```python
from build123d import *

# Parameters (mm, degrees)
F0_W     = 44.45
F0_H     = 44.45
F1_DEPTH = 19.05
F2_R     = 2.38125
F3_DEPTH = 44.451
F2_R_2   = 3.96875
F4_DEPTH = 3.81


with BuildPart() as f1:
    # F0 (on Front) → F1 (new body, symmetric)
    with BuildSketch(Plane.XZ):
        Rectangle(F0_W, F0_H)
    extrude(amount=F1_DEPTH, both=True)

    # F2 (on face) → F3 (cut, through all)
    with BuildSketch(Plane(origin=(0, 0, -22.225), x_dir=(1, 0, 0), z_dir=(0, 0, -1))):
        Circle(F2_R)
    extrude(amount=-F3_DEPTH, mode=Mode.SUBTRACT)

    # F2 (on face) → F4 (cut)
    with BuildSketch(Plane(origin=(0, 0, -22.225), x_dir=(1, 0, 0), z_dir=(0, 0, -1))):
        Circle(F2_R_2)
        Circle(F2_R, mode=Mode.SUBTRACT)
    extrude(amount=-F4_DEPTH, mode=Mode.SUBTRACT)


solid = f1.part
```
For this review, take the finished solid that the model builds, in its own axes (mm). A direction names the side the tool comes from. Round coordinates to 2 decimals unless told otherwise and drop trailing zeros. Loops run counter-clockwise (first coordinate to the right, second up) from the corner with the lowest first, then second, coordinate; pieces in that order, holes last.
(1) Tool access review of faces 4 (the flat face through (2, 2, -18.415)), 5 (the cylindrical face through (-1.89, 1.45, 1.62)): name each direction out of +Z, -Z, +X, -X, +Y, -Y from which nothing blocks a thin tool from reaching the whole face with its end or side.
Returned:
face 4: -Z
face 5: +Z, -Z
(2) We need section A-A (x = 0). Give the boundary of the cut face in (y, z) (3 decimals).
Returned:
outline: (-19.05, -22.225) - (-3.969, -22.225) - (-3.969, -18.415) - (-2.381, -18.415) - (-2.381, 22.225) - (-19.05, 22.225) - close; (2.381, -18.415) - (3.969, -18.415) - (3.969, -22.225) - (19.05, -22.225) - (19.05, 22.225) - (2.381, 22.225) - close
(3) We need section B-B (y = 0). Give the boundary of the cut face in (x, z) (3 decimals), plus the area to 3 significant figures.
Returned:
outline: (-22.225, -22.225) - (-3.969, -22.225) - (-3.969, -18.415) - (-2.381, -18.415) - (-2.381, 22.225) - (-22.225, 22.225) - close; (2.381, -18.415) - (3.969, -18.415) - (3.969, -22.225) - (22.225, -22.225) - (22.225, 22.225) - (2.381, 22.225) - close
area: 1,750 mm2
(4) Wall thickness on line 1 along Y through (x, z) = (0, -8); line 2 along Y through (x, z) = (0, -21); line 3 along X through (y, z) = (0, 5) (3 decimals): over which ranges is each line inside the solid? List them lowest first.
Returned:
line 1: y = -19.05 to -2.38, 2.38 to 19.05
line 2: y = -19.05 to -3.97, 3.97 to 19.05
line 3: x = -22.225 to -2.381, 2.381 to 22.225
(5) Clearance check with flat-ended pins moving along their axes: P1, Ø2.5, axis at x = -2, y = -2, coming from the -Z side (3 decimals); P2, Ø7, axis at x = 0, y = 0, coming from the -Z side (3 decimals). State where each tip first meets the part, or that it passes through.
Returned:
P1: stops at z = -22.225
P2: stops at z = -18.415
(6) Mouldability with a two-part tool opening along X and no side actions: class faces 1 (the flat face through (0, 19.05, 0)), 2 (the cylindrical face through (-0.86, 3.874, -20.347)), 3 (the flat face through (-22.225, 0, 0)) as released by +X, released by -X, zero draft, split by the parting line, or undercut.
Returned:
face 1: zero draft
face 2: undercut
face 3: released by -X
